from build123d import *

# Parameters (mm, degrees)
SKETCH1_W           = 61.6
SKETCH1_H           = 42
BOSS_EXTRUDE1_DEPTH = 5
CUT_EXTRUDE1_DEPTH  = 5
SKETCH3_W           = 61.6
SKETCH3_H           = 6
BOSS_EXTRUDE2_DEPTH = 5


with BuildPart() as part:
    # Sketch1 → Boss-Extrude1 (new body)
    with BuildSketch(Plane.XY):
        with Locations((0, 31)):
            Rectangle(SKETCH1_W, SKETCH1_H)
    extrude(amount=BOSS_EXTRUDE1_DEPTH)

    # Sketch2 → Cut-Extrude1 (cut)
    with BuildSketch(Plane.XY.offset(5)):
        with BuildLine():
            Line((-12.5, 27.5), (-12.5, 32.5))
            ThreePointArc((-12.5, 32.5), (0, 45), (12.5, 32.5))
            Line((12.5, 32.5), (12.5, 27.5))
            ThreePointArc((12.5, 27.5), (0, 15), (-12.5, 27.5))
        make_face()
        with BuildLine():
            Line((-17.1, 45.5), (-17.1, 48))
            ThreePointArc((-17.1, 48), (-15.5, 49.6), (-13.9, 48))
            Line((-13.9, 48), (-13.9, 45.5))
            Line((-13.9, 45.5), (-13.9, 43))
            ThreePointArc((-13.9, 43), (-15.5, 41.4), (-17.1, 43))
            Line((-17.1, 43), (-17.1, 45.5))
        make_face()
        with BuildLine():
            Line((-17.1, 14.5), (-17.1, 12))
            ThreePointArc((-17.1, 12), (-15.5, 10.4), (-13.9, 12))
            Line((-13.9, 12), (-13.9, 14.5))
            Line((-13.9, 14.5), (-13.9, 17))
            ThreePointArc((-13.9, 17), (-15.5, 18.6), (-17.1, 17))
            Line((-17.1, 17), (-17.1, 14.5))
        make_face()
        with BuildLine():
            Line((13.9, 12), (13.9, 14.5))
            Line((13.9, 14.5), (13.9, 17))
            ThreePointArc((13.9, 17), (15.5, 18.6), (17.1, 17))
            Line((17.1, 17), (17.1, 14.5))
            Line((17.1, 14.5), (17.1, 12))
            ThreePointArc((17.1, 12), (15.5, 10.4), (13.9, 12))
        make_face()
        with BuildLine():
            Line((17.1, 45.5), (17.1, 48))
            ThreePointArc((17.1, 48), (15.5, 49.6), (13.9, 48))
            Line((13.9, 48), (13.9, 45.5))
            Line((13.9, 45.5), (13.9, 43))
            ThreePointArc((13.9, 43), (15.5, 41.4), (17.1, 43))
            Line((17.1, 43), (17.1, 45.5))
        make_face()
    extrude(amount=-CUT_EXTRUDE1_DEPTH, mode=Mode.SUBTRACT)

    # Sketch3 → Boss-Extrude2 (add)
    with BuildSketch(Plane.XY.offset(5)):
        with Locations((0, 7)):
            Rectangle(SKETCH3_W, SKETCH3_H)
    extrude(amount=-BOSS_EXTRUDE2_DEPTH)


solid = part.part
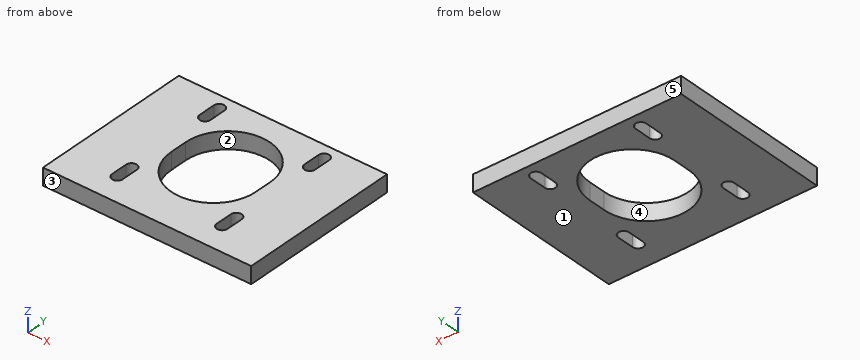
Source: CAD feature listing. Evaluate the final solid. Frame: model axes, mm. Face numbers are marked on the shaded views. A direction names the side the tool comes from. Coordinates: 2 decimals unless noted, no trailing zeros. Order: outer loops, then holes, each group sorted by start corner. A loop starts at its lowest first (then second) coordinate and runs counter-clockwise, first axis right, second up.
Item 1: Cut plane D-D (y = 23). Return loops of the section in (x, z).
Output values:
outline: (-30.8, 0) - (-11.66, 0) - (-11.66, 5) - (-30.8, 5) - close; (11.66, 0) - (30.8, 0) - (30.8, 5) - (11.66, 5) - close
Item 2: Cut plane C-C (z = 2.05). Return loops of the section in (x, y).
Output values:
outline: (-30.8, 4) - (30.8, 4) - (30.8, 52) - (-30.8, 52) - close; hole (-17.1, 12) arc R1.6 ccw to (-13.9, 12) - (-13.9, 17) arc R1.6 ccw to (-17.1, 17) - close; hole (-17.1, 43) arc R1.6 ccw to (-13.9, 43) - (-13.9, 48) arc R1.6 ccw to (-17.1, 48) - close; hole (-12.5, 27.5) arc R12.5 ccw to (12.5, 27.5) - (12.5, 32.5) arc R12.5 ccw to (-12.5, 32.5) - close; hole (13.9, 12) arc R1.6 ccw to (17.1, 12) - (17.1, 17) arc R1.6 ccw to (13.9, 17) - close; hole (13.9, 43) arc R1.6 ccw to (17.1, 43) - (17.1, 48) arc R1.6 ccw to (13.9, 48) - close
Item 3: First-contact query: P1, Ø12, axis at x = 5, y = 13, coming from the -Z side; P2, Ø10, axis at x = -4, y = 25.5, coming from the +Z side. Flat tips, straight axial feed; report the tip coordinate or a pass-through.
Output values:
P1: stops at z = 0
P2: passes through
Item 4: Pull-direction query (Y, two-part tool) for the marked faces 1, 2 and 3; classes: pulls with the +Y half, pulls with the -Y half, needs draft (parallel to the pull), parting line crosses it, or undercut.
Output values:
face 1: needs draft
face 2: undercut
face 3: pulls with the -Y half
Item 5: Material intervals for line 1 (X direction, y = 47.5, z = 3.5); line 2 (X direction, y = 18, z = 1.85); line 3 (Y direction, x = -16.5, z = 2.35), sorted ascending.
Output values:
line 1: x = -30.8 to -17.1, -13.9 to 13.9, 17.1 to 30.8
line 2: x = -30.8 to -16.75, -14.25 to -8.12, 8.12 to 14.25, 16.75 to 30.8
line 3: y = 4 to 10.75, 18.25 to 41.75, 49.25 to 52
Item 6: Set-up query: the marked faces 4 and 5. Return all of +Z, -Z, +X, -X, +Y, -Y with unobstructed straight access to the full face (end or side cutting, diameter ignored); none if empty.
Output values:
face 4: +Z, -Z
face 5: +Z, -Z, +X, -X, +Y
Item 7: Cut plane A-A (x = 0). Return loops of the section in (y, z).
Output values:
outline: (4, 0) - (15, 0) - (15, 5) - (4, 5) - close; (45, 0) - (52, 0) - (52, 5) - (45, 5) - close
Item 8: Cut plane B-B (x = 15.5). Return loops of the section in (y, z), plus the area to 3 significant figures.
Output values:
outline: (4, 0) - (10.4, 0) - (10.4, 5) - (4, 5) - close; (18.6, 0) - (41.4, 0) - (41.4, 5) - (18.6, 5) - close; (49.6, 0) - (52, 0) - (52, 5) - (49.6, 5) - close
area: 158 mm2
